```python
from build123d import *

# Parameters (mm, degrees)
SKETCH1_W           = 116
SKETCH1_H           = 74
BOSS_EXTRUDE1_DEPTH = 15
CUT_EXTRUDE1_DEPTH  = 15
SKETCH4_R           = 4.5
CUT_EXTRUDE2_DEPTH  = 15
SKETCH5_R           = 3
CUT_EXTRUDE3_DEPTH  = 15
SKETCH6_R           = 7.5
CUT_EXTRUDE4_DEPTH  = 6
CUT_EXTRUDE5_DEPTH  = 8
FILLET1_R           = 10
FILLET2_R           = 10


with BuildPart() as part:
    # Sketch1 → Boss-Extrude1 (new body)
    with BuildSketch(Plane(origin=(0, 0, 0), x_dir=(1, 0, 0), z_dir=(0, 1, 0))):
        with Locations((58, 37)):
            Rectangle(SKETCH1_W, SKETCH1_H)
    extrude(amount=BOSS_EXTRUDE1_DEPTH)

    # Sketch2 → Cut-Extrude1 (cut)
    with BuildSketch(Plane(origin=(0, 15, 0), x_dir=(1, 0, 0), z_dir=(0, 1, 0))):
        with BuildLine():
            Line((79.5, 55.5), (36.5, 55.5))
            ThreePointArc((36.5, 55.5), (23.418524548, 50.081475452), (18, 37))
            ThreePointArc((18, 37), (23.418524548, 23.918524548), (36.5, 18.5))
            Line((36.5, 18.5), (79.5, 18.5))
            ThreePointArc((79.5, 18.5), (92.581475452, 23.918524548), (98, 37))
            ThreePointArc((98, 37), (92.581475452, 50.081475452), (79.5, 55.5))
        make_face()
    extrude(amount=-CUT_EXTRUDE1_DEPTH, mode=Mode.SUBTRACT)

    # Sketch4 → Cut-Extrude2 (cut)
    with BuildSketch(Plane(origin=(0, 15, 0), x_dir=(1, 0, 0), z_dir=(0, 1, 0))):
        with Locations(Location((12, 60, 0), (0, 0, 270))):  # turned: the seam where the file's is
            Circle(SKETCH4_R)
        with Locations(Location((12, 14, 0), (0, 0, 270))):  # turned: the seam where the file's is
            Circle(SKETCH4_R)
        with Locations(Location((104, 60, 0), (0, 0, 270))):  # turned: the seam where the file's is
            Circle(SKETCH4_R)
        with Locations(Location((104, 14, 0), (0, 0, 270))):  # turned: the seam where the file's is
            Circle(SKETCH4_R)
    extrude(amount=-CUT_EXTRUDE2_DEPTH, mode=Mode.SUBTRACT)

    # Sketch5 → Cut-Extrude3 (cut)
    with BuildSketch(Plane(origin=(0, 15, 0), x_dir=(1, 0, 0), z_dir=(0, 1, 0))):
        with Locations(Location((9.48, 37, 0), (0, 0, 270))):  # turned: the seam where the file's is
            Circle(SKETCH5_R)
        with Locations(Location((58, 64.27, 0), (0, 0, 270))):  # turned: the seam where the file's is
            Circle(SKETCH5_R)
        with Locations(Location((106.52, 37, 0), (0, 0, 270))):  # turned: the seam where the file's is
            Circle(SKETCH5_R)
        with Locations(Location((58, 9.73, 0), (0, 0, 270))):  # turned: the seam where the file's is
            Circle(SKETCH5_R)
    extrude(amount=-CUT_EXTRUDE3_DEPTH, mode=Mode.SUBTRACT)

    # Sketch6 → Cut-Extrude4 (cut)
    with BuildSketch(Plane(origin=(0, 15, 0), x_dir=(1, 0, 0), z_dir=(0, 1, 0))):
        with Locations(Location((58, 64.27, 0), (0, 0, 270))):  # turned: the seam where the file's is
            Circle(SKETCH6_R)
        with Locations(Location((9.48, 37, 0), (0, 0, 270))):  # turned: the seam where the file's is
            Circle(SKETCH6_R)
        with Locations(Location((106.52, 37, 0), (0, 0, 270))):  # turned: the seam where the file's is
            Circle(SKETCH6_R)
        with Locations(Location((58, 9.73, 0), (0, 0, 270))):  # turned: the seam where the file's is
            Circle(SKETCH6_R)
    extrude(amount=-CUT_EXTRUDE4_DEPTH, mode=Mode.SUBTRACT)

    # Sketch8 → Cut-Extrude5 (cut)
    with BuildSketch(Plane(origin=(0, 0, 0), x_dir=(-1, 0, 0), z_dir=(0, -1, 0))):
        Polygon((-13.979937501, 21.38922735), (-19.38922735, 15.979937501), (-17.409289849, 8.590710151), (-10.020062499, 6.61077265), (-4.61077265, 12.020062499), (-6.590710151, 19.409289849), align=None)
        Polygon((-96.577343391, 15.850676148), (-101.891404254, 21.353547261), (-109.314060863, 19.502871113), (-111.422656609, 12.149323852), (-106.108595746, 6.646452739), (-98.685939137, 8.497128887), align=None)
        Polygon((-102.540331971, 52.490658978), (-96.766885895, 57.509439084), (-98.226553924, 65.018780105), (-105.459668029, 67.509341022), (-111.233114105, 62.490560916), (-109.773446076, 54.981219895), align=None)
        Polygon((-19.275478748, 57.636053655), (-13.590501786, 52.517277407), (-6.315023038, 54.881223752), (-4.724521252, 62.363946345), (-10.409498214, 67.482722593), (-17.684976962, 65.118776248), align=None)
    extrude(amount=-CUT_EXTRUDE5_DEPTH, mode=Mode.SUBTRACT)

    # Fillet1
    fillet1_edges = [part.edges().sort_by_distance(p)[0] for p in [
        (0, 7.5, 0),
        (116, 7.5, 0),
        (116, 7.5, -74),
    ]]
    fillet(fillet1_edges, radius=FILLET1_R)

    # Fillet2
    fillet2_edges = [part.edges().sort_by_distance(p)[0] for p in [
        (0, 7.5, -74),
    ]]
    fillet(fillet2_edges, radius=FILLET2_R)


solid = part.part
```
Geometry check sheet. Reference: the model listing, model coordinates, mm. A direction names the side the tool comes from. Coordinates: 2 decimals unless noted, no trailing zeros. Write each loop counter-clockwise with the first axis right and the second up, starting at its lowest first coordinate (ties: lowest second). Pieces come first, ordered by that corner, then holes. Notation, with made-up numbers: M 38.5,22.25 L 76.5,22.25 A10 cw 76.5,26.25 Z; hole C -40,-30.5 d3. An arc over 180 degrees is marked long. Answer as a JSON object with one key per item and string values.
1. Section check A-A, the plane y = 13.25. Give the number of separate pieces and of enclosed holes in the cut face, plus the area to 3 significant figures.
Answers below:
{"separate pieces": "1", "enclosed holes": "9", "area": "4,870 mm²"}
2. Section check D-D, the plane z = -14. Enter the section's corners in (x, y).
Answers below:
{"outline": "M 0,0 L 5.14,0 L 5.14,8 L 7.5,8 L 7.5,15 L 0,15 Z; M 16.5,8 L 18.86,8 L 18.86,0 L 97.11,0 L 97.11,8 L 99.5,8 L 99.5,15 L 64.17,15 L 64.17,9 L 51.83,9 L 51.83,15 L 16.5,15 Z; M 108.5,8 L 110.89,8 L 110.89,0 L 116,0 L 116,15 L 108.5,15 Z"}
3. Section check C-C, the plane z = -43. Enter the section's corners in (x, y), plus the area to 3 significant figures.
Answers below:
{"outline": "M 0,0 L 19,0 L 19,15 L 13.98,15 L 13.98,9 L 4.98,9 L 4.98,15 L 0,15 Z; M 97,0 L 116,0 L 116,15 L 111.02,15 L 111.02,9 L 102.02,9 L 102.02,15 L 97,15 Z", "area": "462 mm²"}
4. Scan lines: L1, parallel to X at y = 11.35, z = -37; L2, parallel to X at y = 2.25, z = -37; L3, parallel to Z at x = 10, y = 3.75. Record each from-to range of solid material in increasing order.
Answers below:
{"L1": "x = 0 to 1.98, 16.98 to 18, 98 to 99.02, 114.02 to 116", "L2": "x = 0 to 6.48, 12.48 to 18, 98 to 103.52, 109.52 to 116", "L3": "z = -74 to -67.11, -53.68 to -39.95, -34.05 to -20.32, -6.63 to 0"}
5. Go/stop test with flat-tipped pins: pin 1 Ø5 at (x, z) = (58, -9.73) entering from -Y; pin 2 Ø9 at (x, z) = (58, -9.73) entering from +Y; pin 3 Ø7.5 at (x, z) = (106.5, -13.5) entering from -Y. Record where each tip stops, or that it passes through.
Answers below:
{"pin 1": "passes through", "pin 2": "stops at y = 9", "pin 3": "stops at y = 8"}
6. Section check B-B, the plane x = 58. Enter the section's corners in (y, z), plus the area to 3 significant figures.
Answers below:
{"outline": "M 0,-74 L 15,-74 L 15,-71.77 L 9,-71.77 L 9,-67.27 L 0,-67.27 Z; M 0,-61.27 L 9,-61.27 L 9,-56.77 L 15,-56.77 L 15,-55.5 L 0,-55.5 Z; M 0,-18.5 L 15,-18.5 L 15,-17.23 L 9,-17.23 L 9,-12.73 L 0,-12.73 Z; M 0,-6.73 L 9,-6.73 L 9,-2.23 L 15,-2.23 L 15,0 L 0,0 Z", "area": "267 mm²"}
7. Tool access check on faces 4 (the flat face through (58.1, 9, -6.5)), 5 (the flat face through (99.694, 3.944, -54.965)), 6 (the cylindrical face through (107.794, 11.549, -57.581)). Record the directions out of +Z, -Z, +X, -X, +Y, -Y that give a thin tool (end or side, any length) a straight path to the whole face; none if there is none.
Answers below:
{"face 4": "+Y", "face 5": "-Y", "face 6": "+Y, -Y"}
8. Draft check along Z on faces 1 (the flat face through (57, 0, -13)), 2 (the cylindrical face through (2.85, 7.6, -3.01)), 3 (the flat face through (108.803, 3.944, -9.436)). Enter one of: released by +Z, released by -Z, zero draft, split by the parting line, or undercut.
Answers below:
{"face 1": "zero draft", "face 2": "released by +Z", "face 3": "undercut"}
